```python
from build123d import *

# Parameters (mm, degrees)
BOSS_EXTRUDE1_DEPTH                              = 2
BOSS_EXTRUDE2_DEPTH                              = 2
CUT_EXTRUDE1_DEPTH                               = 82.706792863
CBORE_FOR_M2_PAN_HEAD_MACHINE_SCREW1_D           = 2.4
CBORE_FOR_M2_PAN_HEAD_MACHINE_SCREW1_CBORE_D     = 5
CBORE_FOR_M2_PAN_HEAD_MACHINE_SCREW1_CBORE_DEPTH = 1.6
BOSS_EXTRUDE3_START                              = -4
SKETCH8_3_W                                      = 68
SKETCH8_3_H                                      = 58
BOSS_EXTRUDE3_DEPTH                              = 20
SKETCH8_W                                        = 65
SKETCH8_H                                        = 55
CUT_EXTRUDE2_DEPTH                               = 22
SKETCH9_W                                        = 73
SKETCH9_H                                        = 63
CUT_EXTRUDE3_DEPTH                               = 2
BOSS_EXTRUDE4_DEPTH                              = 6
CSK_FOR_M2_FLAT_HEAD_MACHINE_SCREW2_D            = 3
CSK_FOR_M2_FLAT_HEAD_MACHINE_SCREW2_DEPTH        = 6
CSK_FOR_M2_FLAT_HEAD_MACHINE_SCREW2_CSINK_D      = 3.27
CSK_FOR_M2_FLAT_HEAD_MACHINE_SCREW2_CSINK_ANGLE  = 30
CSK_FOR_M2_FLAT_HEAD_MACHINE_SCREW2_TIP          = 0.901290929
SKETCH15_W                                       = 15
SKETCH15_H                                       = 8
CUT_EXTRUDE4_DEPTH                               = 108.53604047
CUT_EXTRUDE5_DEPTH                               = 86.064681273


with BuildPart() as part:
    # Sketch2 → Boss-Extrude1 (new body)
    with BuildSketch(Plane.XY):
        with BuildLine():
            Line((45, -58.5), (45, 58.5))
            ThreePointArc((45, 58.5), (43.681980515, 61.681980515), (40.5, 63))
            Line((40.5, 63), (-40.5, 63))
            ThreePointArc((-40.5, 63), (-43.681980515, 61.681980515), (-45, 58.5))
            Line((-45, 58.5), (-45, -58.5))
            ThreePointArc((-45, -58.5), (-43.681980515, -61.681980515), (-40.5, -63))
            Line((-40.5, -63), (40.5, -63))
            ThreePointArc((40.5, -63), (43.681980515, -61.681980515), (45, -58.5))
        make_face()
    extrude(amount=BOSS_EXTRUDE1_DEPTH)

    # Sketch3 → Boss-Extrude2 (add)
    with BuildSketch(Plane(origin=(0, 0, 0), x_dir=(-1, 0, 0), z_dir=(0, 0, -1))):
        with BuildLine():
            Line((-40.5, -66), (40.5, -66))
            ThreePointArc((40.5, -66), (45.803300859, -63.803300859), (48, -58.5))
            Line((48, -58.5), (48, 58.5))
            ThreePointArc((48, 58.5), (45.803300859, 63.803300859), (40.5, 66))
            Line((40.5, 66), (-40.5, 66))
            ThreePointArc((-40.5, 66), (-45.803300859, 63.803300859), (-48, 58.5))
            Line((-48, 58.5), (-48, -58.5))
            ThreePointArc((-48, -58.5), (-45.803300859, -63.803300859), (-40.5, -66))
        make_face()
    extrude(amount=BOSS_EXTRUDE2_DEPTH)

    # Sketch5 → Cut-Extrude1 (cut, through all)
    with BuildSketch(Plane(origin=(0, 0, -2), x_dir=(-1, 0, 0), z_dir=(0, 0, -1))):
        with BuildLine():
            Line((-36.75, 22), (-33.25, 22))
            ThreePointArc((-33.25, 22), (-31.835786438, 22.585786438), (-31.25, 24))
            Line((-31.25, 24), (-31.25, 52))
            ThreePointArc((-31.25, 52), (-31.835786438, 53.414213562), (-33.25, 54))
            Line((-33.25, 54), (-36.75, 54))
            ThreePointArc((-36.75, 54), (-38.164213562, 53.414213562), (-38.75, 52))
            Line((-38.75, 52), (-38.75, 24))
            ThreePointArc((-38.75, 24), (-38.164213562, 22.585786438), (-36.75, 22))
        make_face()
        with BuildLine():
            Line((-21.25, 24), (-21.25, 52))
            ThreePointArc((-21.25, 52), (-20.664213562, 53.414213562), (-19.25, 54))
            Line((-19.25, 54), (-15.75, 54))
            ThreePointArc((-15.75, 54), (-14.335786438, 53.414213562), (-13.75, 52))
            Line((-13.75, 52), (-13.75, 24))
            ThreePointArc((-13.75, 24), (-14.335786438, 22.585786438), (-15.75, 22))
            Line((-15.75, 22), (-19.25, 22))
            ThreePointArc((-19.25, 22), (-20.664213562, 22.585786438), (-21.25, 24))
        make_face()
        with BuildLine():
            Line((-3.75, 24), (-3.75, 52))
            ThreePointArc((-3.75, 52), (-3.164213562, 53.414213562), (-1.75, 54))
            Line((-1.75, 54), (1.75, 54))
            ThreePointArc((1.75, 54), (3.164213562, 53.414213562), (3.75, 52))
            Line((3.75, 52), (3.75, 24))
            ThreePointArc((3.75, 24), (3.164213562, 22.585786438), (1.75, 22))
            Line((1.75, 22), (-1.75, 22))
            ThreePointArc((-1.75, 22), (-3.164213562, 22.585786438), (-3.75, 24))
        make_face()
        with BuildLine():
            Line((13.75, 24), (13.75, 52))
            ThreePointArc((13.75, 52), (14.335786438, 53.414213562), (15.75, 54))
            Line((15.75, 54), (19.25, 54))
            ThreePointArc((19.25, 54), (20.664213562, 53.414213562), (21.25, 52))
            Line((21.25, 52), (21.25, 24))
            ThreePointArc((21.25, 24), (20.664213562, 22.585786438), (19.25, 22))
            Line((19.25, 22), (15.75, 22))
            ThreePointArc((15.75, 22), (14.335786438, 22.585786438), (13.75, 24))
        make_face()
        with BuildLine():
            Line((31.25, 24), (31.25, 52))
            ThreePointArc((31.25, 52), (31.835786438, 53.414213562), (33.25, 54))
            Line((33.25, 54), (36.75, 54))
            ThreePointArc((36.75, 54), (38.164213562, 53.414213562), (38.75, 52))
            Line((38.75, 52), (38.75, 24))
            ThreePointArc((38.75, 24), (38.164213562, 22.585786438), (36.75, 22))
            Line((36.75, 22), (33.25, 22))
            ThreePointArc((33.25, 22), (31.835786438, 22.585786438), (31.25, 24))
        make_face()
    extrude(amount=-CUT_EXTRUDE1_DEPTH, mode=Mode.SUBTRACT)

    # CBORE for M2 Pan Head Machine Screw1 (through all)
    with Locations(Plane(origin=(0, 0, -2), x_dir=(-1, 0, 0), z_dir=(0, 0, -1))):
        with Locations((-42.1, 60.1), (42.1, 60.1), (-42.1, -60.1), (42.1, -60.1)):
            CounterBoreHole(CBORE_FOR_M2_PAN_HEAD_MACHINE_SCREW1_D / 2, CBORE_FOR_M2_PAN_HEAD_MACHINE_SCREW1_CBORE_D / 2, CBORE_FOR_M2_PAN_HEAD_MACHINE_SCREW1_CBORE_DEPTH)

    # Sketch8<3> → Boss-Extrude3 (add)
    with BuildSketch(Plane(origin=(0, 0, -2), x_dir=(-1, 0, 0), z_dir=(0, 0, -1)).offset(BOSS_EXTRUDE3_START)):
        with Locations((0, -20.5)):
            Rectangle(SKETCH8_3_W, SKETCH8_3_H)
    extrude(amount=-BOSS_EXTRUDE3_DEPTH)

    # Sketch8 → Cut-Extrude2 (cut)
    with BuildSketch(Plane(origin=(0, 0, -2), x_dir=(-1, 0, 0), z_dir=(0, 0, -1))):
        with Locations((0, -20.5)):
            Rectangle(SKETCH8_W, SKETCH8_H)
    extrude(amount=-CUT_EXTRUDE2_DEPTH, mode=Mode.SUBTRACT)

    # Sketch9 → Cut-Extrude3 (cut)
    with BuildSketch(Plane(origin=(0, 0, -2), x_dir=(-1, 0, 0), z_dir=(0, 0, -1))):
        with Locations((0, -20.5)):
            Rectangle(SKETCH9_W, SKETCH9_H)
    extrude(amount=-CUT_EXTRUDE3_DEPTH, mode=Mode.SUBTRACT)

    # Sketch10 → Boss-Extrude4 (add)
    with BuildSketch(Plane.XY.offset(2)):
        with BuildLine():
            Line((32.5, 7), (32, 7))
            ThreePointArc((32, 7), (35.767766953, 10.267766953), (32.5, 6.5))
            Line((32.5, 6.5), (32.5, 7))
        make_face()
        with BuildLine():
            Line((-32.5, 7), (-32.5, 6.5))
            ThreePointArc((-32.5, 6.5), (-35.767766953, 10.267766953), (-32, 7))
            Line((-32, 7), (-32.5, 7))
        make_face()
        with BuildLine():
            Line((-32.5, -48), (-32, -48))
            ThreePointArc((-32, -48), (-35.767766953, -51.267766953), (-32.5, -47.5))
            Line((-32.5, -47.5), (-32.5, -48))
        make_face()
        with BuildLine():
            Line((32.5, -48), (32.5, -47.5))
            ThreePointArc((32.5, -47.5), (35.767766953, -51.267766953), (32, -48))
            Line((32, -48), (32.5, -48))
        make_face()
    extrude(amount=BOSS_EXTRUDE4_DEPTH)

    # CSK for M2 Flat Head Machine Screw2
    with Locations(Plane(origin=(0, 0, 0), x_dir=(-1, 0, 0), z_dir=(0, 0, -1))):
        with Locations((-34, 8.5), (34, 8.5), (-34, -49.5), (34, -49.5)):
            CounterSinkHole(CSK_FOR_M2_FLAT_HEAD_MACHINE_SCREW2_D / 2, CSK_FOR_M2_FLAT_HEAD_MACHINE_SCREW2_CSINK_D / 2, depth=CSK_FOR_M2_FLAT_HEAD_MACHINE_SCREW2_DEPTH, counter_sink_angle=CSK_FOR_M2_FLAT_HEAD_MACHINE_SCREW2_CSINK_ANGLE)
            with Locations((0, 0, -(CSK_FOR_M2_FLAT_HEAD_MACHINE_SCREW2_DEPTH + CSK_FOR_M2_FLAT_HEAD_MACHINE_SCREW2_TIP / 2))):  # 118° drill point
                Cone(0, CSK_FOR_M2_FLAT_HEAD_MACHINE_SCREW2_D / 2, CSK_FOR_M2_FLAT_HEAD_MACHINE_SCREW2_TIP, mode=Mode.SUBTRACT)

    # Sketch15 → Cut-Extrude4 (cut, through all)
    with BuildSketch(Plane(origin=(34, 0, 0), x_dir=(0, 0, -1), z_dir=(1, 0, 0))):
        with Locations((-9.5, -20.5)):
            Rectangle(SKETCH15_W, SKETCH15_H)
    extrude(amount=-CUT_EXTRUDE4_DEPTH, mode=Mode.SUBTRACT)

    # Sketch16 → Cut-Extrude5 (cut, through all)
    with BuildSketch(Plane(origin=(0, 0, -2), x_dir=(-1, 0, 0), z_dir=(0, 0, -1))):
        with BuildLine():
            Line((2.515812527, -57.4), (-2.515812527, -57.4))
            ThreePointArc((-2.515812527, -57.4), (-2.727890225, -57.352794711), (-2.899923167, -57.2200922))
            Line((-2.899923167, -57.2200922), (-3.88411064, -56.039067232))
            ThreePointArc((-3.88411064, -56.039067232), (-3.970135789, -55.889187664), (-4, -55.718975032))
            Line((-4, -55.718975032), (-4, -54.9))
            ThreePointArc((-4, -54.9), (-3.853553391, -54.546446609), (-3.5, -54.4))
            Line((-3.5, -54.4), (3.5, -54.4))
            ThreePointArc((3.5, -54.4), (3.853553391, -54.546446609), (4, -54.9))
            Line((4, -54.9), (4, -55.718975032))
            ThreePointArc((4, -55.718975032), (3.970135789, -55.889187664), (3.88411064, -56.039067232))
            Line((3.88411064, -56.039067232), (2.899923167, -57.2200922))
            ThreePointArc((2.899923167, -57.2200922), (2.727890225, -57.352794711), (2.515812527, -57.4))
        make_face()
    extrude(amount=-CUT_EXTRUDE5_DEPTH, mode=Mode.SUBTRACT)


solid = part.part
```
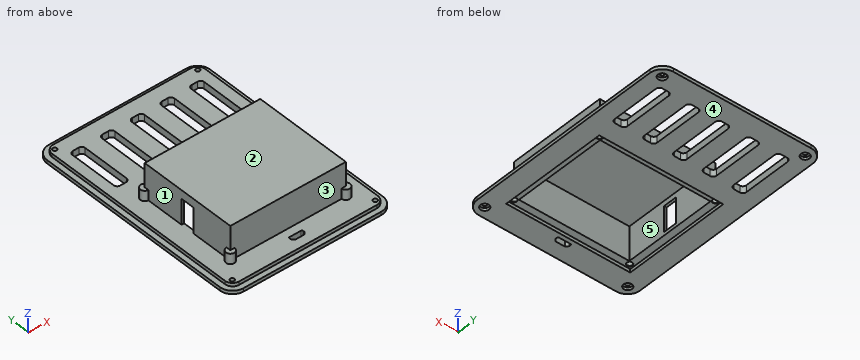
Can you work these out from the model? Positions are in its coordinate system, mm. Face numbers are marked on the shaded views. A direction names the side the tool comes from. Round coordinates to 2 decimals unless told otherwise and drop trailing zeros. Loops run counter-clockwise (first coordinate to the right, second up) from the corner with the lowest first, then second, coordinate; pieces in that order, holes last.
Item 1: Suppose I cut it at A-A, the plane y = 30.5. Write out the boundary of the cut face in (x, z).
Item 2: Suppose I cut it at C-C, the plane x = 26.5. Write out the boundary of the cut face in (y, z).
Item 3: Will these pins go through, and if not, where does the flat tip stop? pin 1 Ø5 at (x, z) = (25.5, 3.5) entering from -Y; pin 2 Ø10 at (x, z) = (0.5, 5.5) entering from +Y; pin 3 Ø12 at (x, z) = (-19.5, 17.5) entering from +Y; pin 4 Ø2 at (x, y) = (-2, 32) entering from +Z.
Item 4: Suppose I cut it at B-B, the plane y = -35.5. Write out the boundary of the cut face in (x, z).
Item 5: If we mould it in two halves opening along X, with no side actions, what happens to the marked faces 1, 2 and 3? For each: +X half, -X half, draft (parallel to the pull), parting line (faces both ways), or undercut.
Item 6: Which directions (+Z, -Z, +X, -X, +Y, -Y) give clear straight access to the entire face, cutting with the end or side of a thin tool? Please do the marked faces 4 and 5.
Item 7: Please list where these lines run through material, in increasing order: L1, parallel to Y at x = 23, z = 15; L2, parallel to Z at x = -33, y = -21.5; L3, parallel to Y at x = -42.1, z = -0.95.
Reported:
1. outline: (-48, -2) - (-38.75, -2) - (-38.75, 2) - (-45, 2) - (-45, 0) - (-48, 0) - close; (-31.25, -2) - (-21.25, -2) - (-21.25, 2) - (-31.25, 2) - close; (-13.75, -2) - (-3.75, -2) - (-3.75, 2) - (-13.75, 2) - close; (3.75, -2) - (13.75, -2) - (13.75, 2) - (3.75, 2) - close; (21.25, -2) - (31.25, -2) - (31.25, 2) - (21.25, 2) - close; (38.75, -2) - (48, -2) - (48, 0) - (45, 0) - (45, 2) - (38.75, 2) - close
2. outline: (-66, -2) - (-52, -2) - (-52, 0) - (-48, 0) - (-48, 20) - (7, 20) - (7, 0) - (11, 0) - (11, -2) - (66, -2) - (66, 0) - (63, 0) - (63, 2) - (8.5, 2) - (8.5, 22) - (-49.5, 22) - (-49.5, 2) - (-63, 2) - (-63, 0) - (-66, 0) - close
3. pin 1: stops at y = -63
3. pin 2: stops at y = 63
3. pin 3: stops at y = 8.5
3. pin 4: passes through
4. outline: (-48, -2) - (-36.5, -2) - (-36.5, 0) - (-32.5, 0) - (-32.5, 20) - (32.5, 20) - (32.5, 0) - (36.5, 0) - (36.5, -2) - (48, -2) - (48, 0) - (45, 0) - (45, 2) - (34, 2) - (34, 22) - (-34, 22) - (-34, 2) - (-45, 2) - (-45, 0) - (-48, 0) - close
5. face 1: -X half
5. face 2: draft
5. face 3: undercut
6. face 4: -Z, +X, -X, +Y, -Y
6. face 5: -Z
7. L1: y = -49.5 to -48, 7 to 8.5
7. L2: z = 0 to 2, 17 to 22
7. L3: y = -65.83 to -62.6, -57.6 to 57.6, 62.6 to 65.83
